The model under review builds one solid part; all positions refer to its coordinate system, in mm. A direction names the side the tool comes from. Round coordinates to 2 decimals unless told otherwise and drop trailing zeros. Write each loop counter-clockwise with the first axis right and the second up, starting at its lowest first coordinate (ties: lowest second). Pieces come first, ordered by that corner, then holes. Notation, with made-up numbers: (-26.75, 47) -> (19.25, 47) arc R16 cw to (19.25, 63) -> close; hole circle Ø2 at (54.5, -13). An arc over 180 degrees is marked (long way). Use CSV: the item, a comma, the result in double quotes. Start each with the question number.
1) Mouldability with a two-part tool opening along Y and no side actions: class faces 5 (the face through (-162, -9, 50)), 6 (the face through (-102, -121.726, -2)), 7 (the face through (-154.539, -111.077, -9.26)), 8 (the face through (-47.93, -110.96, -9.26)) as released by +Y, released by -Y, zero draft, split by the parting line, or undercut.
2) Take a section at A-A, the plane x = -121.5. Give the boundary of the cut face in (y, z), then the cut area to 3 significant figures.
3) Wall thickness on probe 1 along Y at (x, z) = (-88.5, 14.5); probe 2 along X at (y, z) = (13, 36); probe 3 along Z at (x, y) = (-123, 76): over which ranges is each line inside the solid? List them lowest first. Write a range as [from, to].
4) Machinability: for faces 1 (the face through (-102, -111.726, 25)), 2 (the face through (-149.794, -16, -4)), 3 (the face through (-150, -16, 0)), 4 (the face through (-48.049, 77.645, -9.26)), which of the approach directions +Z, -Z, +X, -X, +Y, -Y give a long, thin tool a straight path to every point of the face, cutting with its end or side? Answer none if there is none.
5) Take a section at B-B, the plane y = 57. Give the boundary of the cut face in (x, z).
6) For pin 1 Ø1.2 at (x, z) = (-95, -9) entering from -Y; pin 2 Ø8 at (y, z) = (-7.5, 6.5) entering from +X; pin 3 Ø15 at (x, z) = (-93.5, 21.5) entering from +Y; pin 4 Ø7 at (y, z) = (-54, -6) entering from +X, all flat-tipped, find the tip position at first contact; note any pin that passes through.
7) Take a section at C-C, the plane z = 12.5. Give the boundary of the cut face in (x, y), then the cut area to 3 significant figures.
from build123d import *

# Parameters (mm, degrees)
F0_W     = 135
F0_H     = 190
F0_W_2   = 119
F0_H_2   = 174
F1_DEPTH = 50
F0_W_3   = 155
F0_H_3   = 210
F2_DEPTH = 10
F3_SIZE  = 5
F5_DEPTH = 1.5
F6_W     = 101.5
F6_H     = 170
F7_DEPTH = 60.001


# Not quite as in the source:
# - a feature names something its author has since deleted; it is built from what else it names


with BuildPart() as f1:
    # F0 (on Top) → F1 (new body)
    with BuildSketch(Plane.XY):
        with Locations((-101.2938845903, -16.7257675529)):
            Rectangle(F0_W, F0_H)
        with Locations((-101.2938845903, -16.7257675529)):
            Rectangle(F0_W_2, F0_H_2, mode=Mode.SUBTRACT)
    extrude(amount=F1_DEPTH)

    # F0 (on Top) → F2 (join)
    with BuildSketch(Plane.XY):
        with Locations((-101.2938845903, -16.7257675529)):
            Rectangle(F0_W_3, F0_H_3)
        with Locations((-101.2938845903, -16.7257675529)):
            Rectangle(F0_W, F0_H, mode=Mode.SUBTRACT)
        with Locations((-101.2938845903, -16.7257675529)):
            Rectangle(F0_W, F0_H)
        with Locations((-101.2938845903, -16.7257675529)):
            Rectangle(F0_W_2, F0_H_2, mode=Mode.SUBTRACT)
        with Locations((-101.2938845903, -16.7257675529)):
            Rectangle(F0_W_2, F0_H_2)
    extrude(amount=-F2_DEPTH)

    # F3
    f3_edges = [f1.edges().sort_by_distance(p)[0] for p in [
        (-101.293885, 88.274232, -10),
        (-178.793885, -16.725768, -10),
        (-101.293885, -121.725768, -10),
        (-23.793885, -16.725768, -10),
    ]]
    chamfer(f3_edges, length=F3_SIZE)

    # F4 (on face) → F5 (cut)
    with BuildSketch(Plane(origin=(0, 0, -10), x_dir=(1, 0, 0), z_dir=(0, 0, -1))):
        with BuildLine():
            Line((-53.2938845903, 113.2159726396), (-149.2938845903, 113.2159726396))
            ThreePointArc((-149.2938845903, 113.2159726396), (-154.5971854492, 111.0192734985), (-156.7938845903, 105.7159726396))
            Line((-156.7938845903, 105.7159726396), (-156.7938845903, -72.2840273604))
            ThreePointArc((-156.7938845903, -72.2840273604), (-154.5971854492, -77.5873282193), (-149.2938845903, -79.7840273604))
            Line((-149.2938845903, -79.7840273604), (-53.2938845903, -79.7840273604))
            ThreePointArc((-53.2938845903, -79.7840273604), (-47.9905837314, -77.5873282193), (-45.7938845903, -72.2840273604))
            Line((-45.7938845903, -72.2840273604), (-45.7938845903, 105.7159726396))
            ThreePointArc((-45.7938845903, 105.7159726396), (-47.9905837314, 111.0192734985), (-53.2938845903, 113.2159726396))
        make_face()
    extrude(amount=-F5_DEPTH, mode=Mode.SUBTRACT)

    # F6 (on face) → F7 (cut, through all)
    with BuildSketch(Plane(origin=(0, 0, -10), x_dir=(1, 0, 0), z_dir=(0, 0, -1))):
        with Locations((-99.0438845903, 17.2159726396)):
            Rectangle(F6_W, F6_H)
    extrude(amount=-F7_DEPTH, mode=Mode.SUBTRACT)


solid = f1.part
Values found:
1,face 5,"zero draft"
1,face 6,"released by -Y"
1,face 7,"undercut"
1,face 8,"undercut"
2,outline,"(-121.73, -5) -> (-116.73, -10) -> (-113.22, -10) -> (-113.22, -8.5) -> (-102.22, -8.5) -> (-102.22, 0) -> (-103.73, 0) -> (-103.73, 50) -> (-111.73, 50) -> (-111.73, 0) -> (-121.73, 0) -> close; (67.78, -8.5) -> (79.78, -8.5) -> (79.78, -10) -> (83.27, -10) -> (88.27, -5) -> (88.27, 0) -> (78.27, 0) -> (78.27, 50) -> (70.27, 50) -> (70.27, 0) -> (67.78, 0) -> close"
2,area,"1,140 mm²"
3,probe 1,"[-111.73, -103.73], [70.27, 78.27]"
3,probe 2,"[-168.79, -160.79], [-41.79, -33.79]"
3,probe 3,"[-8.5, 50]"
4,face 1,"+Z, +X, -X, -Y"
4,face 2,"+Z, -Z"
4,face 3,"+Z"
4,face 4,"-Z"
5,outline,"(-178.79, -5) -> (-173.79, -10) -> (-156.79, -10) -> (-156.79, -8.5) -> (-149.79, -8.5) -> (-149.79, 0) -> (-160.79, 0) -> (-160.79, 50) -> (-168.79, 50) -> (-168.79, 0) -> (-178.79, 0) -> close; (-48.29, -8.5) -> (-45.79, -8.5) -> (-45.79, -10) -> (-28.79, -10) -> (-23.79, -5) -> (-23.79, 0) -> (-33.79, 0) -> (-33.79, 50) -> (-41.79, 50) -> (-41.79, 0) -> (-48.29, 0) -> close"
6,pin 1,"y = -118.33"
6,pin 2,"x = -33.79"
6,pin 3,"y = 78.27"
6,pin 4,"x = -23.79"
7,outline,"(-168.79, -111.73) -> (-33.79, -111.73) -> (-33.79, 78.27) -> (-168.79, 78.27) -> close; hole (-160.79, -103.73) -> (-41.79, -103.73) -> (-41.79, 70.27) -> (-160.79, 70.27) -> close"
7,area,"4,940 mm²"
